Can you work these out from the model? Positions are in its coordinate system, mm. Face numbers are marked on the shaded views. A direction names the side the tool comes from. Give positions to 0.01 mm unless a question says otherwise; leave off trailing zeros. Order: outer loops, then holes, each group sorted by start corner. A loop starts at its lowest first (then second) coordinate and runs counter-clockwise, first axis right, second up.
Item 1: I want a section at B-B, the plane x = -2. Write out the boundary of the cut face in (y, z).
Item 2: I want a section at A-A, the plane z = 6.5. Write out the boundary of the cut face in (x, y), then the cut area to 3 significant figures.
Item 3: I want a section at C-C, the plane y = -11.25. Write out the boundary of the cut face in (x, z), then the cut area to 3 significant figures.
Item 4: I want a section at D-D, the plane z = 0. Count the separate pieces of the cut face and the enclosed holes in it, then the cut area to 3 significant figures.
Item 5: Which directions (+Z, -Z, +X, -X, +Y, -Y) give clear straight access to the entire face, cutting with the end or side of a thin tool? Please do the marked faces 5 and 6.
Item 6: I'm going to push flat-ended pins straight in: pin 1 Ø2.5 at (x, z) = (13, -0.5) entering from -Y; pin 2 Ø3 at (x, z) = (31.75, 0) entering from +Y; pin 3 Ø1.9 at (y, z) = (-10, -1.5) entering from -X; pin 4 Ø1 at (y, z) = (-9, -3.5) entering from +X. Where does each tip first touch, or does it pass through?
Item 7: If we mould it in two halves opening along X, with no side actions, what happens to the marked faces 1, 2, 3 and 4? For each: +X half, -X half, draft (parallel to the pull), parting line (faces both ways), or undercut.
Item 8: If I drill on line 1 along X through (y, z) = (-9.25, 0); line 2 along X through (y, z) = (-4.5, 0); line 3 along X through (y, z) = (-10.5, -5), over which ranges is the centre line in solid material (lowest first)?
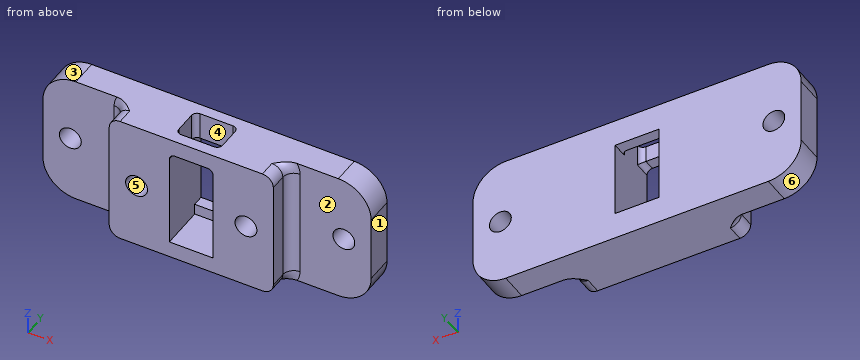
```python
from build123d import *

# Parameters (mm, degrees)
SKETCH1_W           = 38.1
SKETCH1_H           = 30.48
SKETCH1_R           = 2.54
SKETCH1_W_2         = 10.16
SKETCH1_H_2         = 22.86
BOSS_EXTRUDE1_DEPTH = 12.7
SKETCH2_W           = 10.16
SKETCH2_H           = 2.54
BOSS_EXTRUDE2_DEPTH = 2.54
SKETCH3_W           = 10.16
SKETCH3_H           = 2.54
BOSS_EXTRUDE3_DEPTH = 2.54
FILLET1_R           = 2.54
SKETCH4_W           = 10.16
SKETCH4_H           = 7.62
CUT_EXTRUDE1_DEPTH  = 36.149415358
FILLET2_R           = 1.27
BOSS_EXTRUDE4_START = -6.35
SKETCH5_R           = 2.54
BOSS_EXTRUDE4_DEPTH = 6.35
SKETCH6_R           = 2.54
CUT_EXTRUDE2_DEPTH  = 43.955297694
FILLET3_R           = 7.62
FILLET4_R           = 2.54


with BuildPart() as part:
    # Sketch1 → Boss-Extrude1 (new body)
    with BuildSketch(Plane(origin=(0, 0, 0), x_dir=(1, 0, 0), z_dir=(0, 1, 0))):
        Rectangle(SKETCH1_W, SKETCH1_H)
        with Locations(Location((12.7, 0, 0), (0, 0, 270))):
            Circle(SKETCH1_R, mode=Mode.SUBTRACT)
        with Locations(Location((-12.7, 0, 0), (0, 0, 270))):
            Circle(SKETCH1_R, mode=Mode.SUBTRACT)
        Rectangle(SKETCH1_W_2, SKETCH1_H_2, mode=Mode.SUBTRACT)
    extrude(amount=-BOSS_EXTRUDE1_DEPTH)

    # Sketch2 → Boss-Extrude2 (add)
    with BuildSketch(Plane.XY.offset(-11.43)):
        with Locations((0, -1.27)):
            Rectangle(SKETCH2_W, SKETCH2_H)
    extrude(amount=BOSS_EXTRUDE2_DEPTH)

    # Sketch3 → Boss-Extrude3 (add)
    with BuildSketch(Plane(origin=(0, 0, 11.43), x_dir=(-1, 0, 0), z_dir=(0, 0, -1))):
        with Locations((0, -1.27)):
            Rectangle(SKETCH3_W, SKETCH3_H)
    extrude(amount=BOSS_EXTRUDE3_DEPTH)

    # Fillet1
    fillet1_edges = [part.edges().sort_by_distance(p)[0] for p in [
        (19.05, -6.35, 15.24),
        (-19.05, -6.35, 15.24),
        (-19.05, -6.35, -15.24),
        (19.05, -6.35, -15.24),
    ]]
    fillet(fillet1_edges, radius=FILLET1_R)

    # Sketch4 → Cut-Extrude1 (cut, through all)
    with BuildSketch(Plane(origin=(0, 0, 11.43), x_dir=(-1, 0, 0), z_dir=(0, 0, -1))):
        with Locations((0, -6.35)):
            Rectangle(SKETCH4_W, SKETCH4_H)
    extrude(amount=-CUT_EXTRUDE1_DEPTH, mode=Mode.SUBTRACT)

    # Fillet2
    fillet2_edges = [part.edges().sort_by_distance(p)[0] for p in [
        (-5.08, -11.43, 11.43),
        (5.08, -11.43, 11.43),
        (-5.08, -2.54, 12.065),
        (5.08, -2.54, 12.065),
        (5.08, -10.16, 13.335),
        (-5.08, -10.16, 13.335),
    ]]
    fillet(fillet2_edges, radius=FILLET2_R)

    # Sketch5 → Boss-Extrude4 (add)
    with BuildSketch(Plane(origin=(0, 0, 0), x_dir=(1, 0, 0), z_dir=(0, 1, 0)).offset(BOSS_EXTRUDE4_START)):
        with BuildLine():
            Line((-16.51, 15.24), (-38.1, 15.24))
            Line((-38.1, 15.24), (-38.1, -15.24))
            Line((-38.1, -15.24), (-16.51, -15.24))
            ThreePointArc((-16.51, -15.24), (-18.306051224, -14.496051224), (-19.05, -12.7))
            Line((-19.05, -12.7), (-19.05, 12.7))
            ThreePointArc((-19.05, 12.7), (-18.306051224, 14.496051224), (-16.51, 15.24))
        make_face()
        with BuildLine():
            Line((38.1, 15.24), (16.51, 15.24))
            ThreePointArc((16.51, 15.24), (18.306051224, 14.496051224), (19.05, 12.7))
            Line((19.05, 12.7), (19.05, -12.7))
            ThreePointArc((19.05, -12.7), (18.306051224, -14.496051224), (16.51, -15.24))
            Line((16.51, -15.24), (38.1, -15.24))
            Line((38.1, -15.24), (38.1, 15.24))
        make_face()
        with Locations(Location((12.7, 0, 0), (0, 0, 270))):
            Circle(SKETCH5_R)
        with Locations(Location((-12.7, 0, 0), (0, 0, 270))):
            Circle(SKETCH5_R)
    extrude(amount=BOSS_EXTRUDE4_DEPTH)

    # Sketch6 → Cut-Extrude2 (cut, through all)
    with BuildSketch(Plane(origin=(0, 0, 0), x_dir=(1, 0, 0), z_dir=(0, 1, 0))):
        with Locations(Location((-31.75, 0, 0), (0, 0, 270))):
            Circle(SKETCH6_R)
        with Locations(Location((31.75, 0, 0), (0, 0, 270))):
            Circle(SKETCH6_R)
    extrude(amount=-CUT_EXTRUDE2_DEPTH, mode=Mode.SUBTRACT)

    # Fillet3
    fillet3_edges = [part.edges().sort_by_distance(p)[0] for p in [
        (38.1, -3.175, 15.24),
        (-38.1, -3.175, 15.24),
        (-38.1, -3.175, -15.24),
        (38.1, -3.175, -15.24),
    ]]
    fillet(fillet3_edges, radius=FILLET3_R)

    # Fillet4
    # the kernel refuses this fillet: 2.54 mm, written as the material it adds along each edge
    with BuildSketch(Plane(origin=(-16.51, -6.35, -12.7), x_dir=(-1, 0, 0), z_dir=(0, 0, 1))) as fillet4_piece_1_section:
        with BuildLine():
            CenterArc((2.54 + FILLET4_R, FILLET4_R), FILLET4_R, 180, 90)
            Line((2.54, FILLET4_R), (2.54, 0))
            Line((2.54, 0), (2.54 + FILLET4_R, 0))
        make_face()
    fillet4_piece_1 = revolve(axis=Axis((-16.51, -6.35, -12.7), (0, -1, 0)), revolution_arc=233.296989237, mode=Mode.PRIVATE)
    fillet4_piece_1 = split(fillet4_piece_1, bisect_by=Plane(origin=(-19.608229137, -6.77494251, -15.24), z_dir=(0, 0, 1)), keep=Keep.TOP, mode=Mode.PRIVATE)
    add(fillet4_piece_1)
    with BuildSketch(Plane(origin=(16.51, -6.35, 12.7), x_dir=(1, 0, 0), z_dir=(0, 0, -1))) as fillet4_piece_2_section:
        with BuildLine():
            CenterArc((2.54 + FILLET4_R, FILLET4_R), FILLET4_R, 180, 90)
            Line((2.54, FILLET4_R), (2.54, 0))
            Line((2.54, 0), (2.54 + FILLET4_R, 0))
        make_face()
    fillet4_piece_2 = revolve(axis=Axis((16.51, -6.35, 12.7), (0, -1, 0)), revolution_arc=233.296989237, mode=Mode.PRIVATE)
    fillet4_piece_2 = split(fillet4_piece_2, bisect_by=Plane(origin=(19.608229137, -6.77494251, 15.24), z_dir=(0, 0, -1)), keep=Keep.TOP, mode=Mode.PRIVATE)
    add(fillet4_piece_2)
    with BuildSketch(Plane(origin=(-16.51, -6.35, 12.7), x_dir=(0.5976672776328222, 0, -0.8017442392976523), z_dir=(-0.8017442392976523, 0, -0.5976672776328222))) as fillet4_piece_3_section:
        with BuildLine():
            CenterArc((2.54 + FILLET4_R, FILLET4_R), FILLET4_R, 180, 90)
            Line((2.54, FILLET4_R), (2.54, 0))
            Line((2.54, 0), (2.54 + FILLET4_R, 0))
        make_face()
    fillet4_piece_3 = revolve(axis=Axis((-16.51, -6.35, 12.7), (0, -1, 0)), revolution_arc=233.296989237, mode=Mode.PRIVATE)
    fillet4_piece_3 = split(fillet4_piece_3, bisect_by=Plane(origin=(-18.414845025, -7.141535935, 15.24), z_dir=(0, 0, -1)), keep=Keep.TOP, mode=Mode.PRIVATE)
    add(fillet4_piece_3)
    with BuildSketch(Plane(origin=(-19.05, -6.35, 12.7), x_dir=(-1, 0, 0), z_dir=(0, 0, -1)), Plane(origin=(19.05, -6.35, -12.7), x_dir=(1, 0, 0), z_dir=(0, 0, 1))) as fillet4_piece_4:
        with BuildLine():
            CenterArc((FILLET4_R, -FILLET4_R), FILLET4_R, 90, 90)
            Line((0, -FILLET4_R), (0, 0))
            Line((0, 0), (FILLET4_R, 0))
        make_face()
    extrude(amount=25.4)
    with BuildSketch(Plane(origin=(16.51, -6.35, -12.7), x_dir=(-0.5976672776328322, 0, 0.8017442392976448), z_dir=(0.8017442392976448, 0, 0.5976672776328322))) as fillet4_piece_5_section:
        with BuildLine():
            CenterArc((2.54 + FILLET4_R, FILLET4_R), FILLET4_R, 180, 90)
            Line((2.54, FILLET4_R), (2.54, 0))
            Line((2.54, 0), (2.54 + FILLET4_R, 0))
        make_face()
    fillet4_piece_5 = revolve(axis=Axis((16.51, -6.35, -12.7), (0, -1, 0)), revolution_arc=233.296989237, mode=Mode.PRIVATE)
    fillet4_piece_5 = split(fillet4_piece_5, bisect_by=Plane(origin=(18.414845035, -7.141535946, -15.24), z_dir=(0, 0, 1)), keep=Keep.TOP, mode=Mode.PRIVATE)
    add(fillet4_piece_5)


solid = part.part
```
Results list:
1. outline: (-12.7, -15.24) - (0, -15.24) - (0, -8.89) - (-2.54, -8.89) - (-2.54, -11.43) - (-12.7, -11.43) - close; (-12.7, 11.43) - (-10.16, 11.43) - (-10.16, 15.24) - (-12.7, 15.24) - close; (-2.54, 8.89) - (0, 8.89) - (0, 15.24) - (-2.54, 15.24) - close
2. outline: (-38.1, -6.35) - (-21.59, -6.35) arc R2.54 cw to (-19.05, -8.89) - (-19.05, -12.7) - (-5.08, -12.7) - (-5.08, 0) - (-38.1, 0) - close; (5.08, -12.7) - (19.05, -12.7) - (19.05, -8.89) arc R2.54 cw to (21.59, -6.35) - (38.1, -6.35) - (38.1, 0) - (5.08, 0) - close
2. area: 600 mm2
3. outline: (-19.05, -12.7) arc R2.54 ccw to (-16.51, -15.24) - (16.51, -15.24) arc R2.54 ccw to (19.05, -12.7) - (19.05, 12.7) arc R2.54 ccw to (16.51, 15.24) - (-16.51, 15.24) arc R2.54 ccw to (-19.05, 12.7) - close; hole circle Ø5.08 at (-12.7, 0); hole (-5.08, -11.43) - (5.08, -11.43) - (5.08, 10.16) arc R1.27 ccw to (3.81, 11.43) - (-3.81, 11.43) arc R1.27 ccw to (-5.08, 10.16) - close; hole circle Ø5.08 at (12.7, 0)
3. area: 884 mm2
4. separate pieces: 4
4. enclosed holes: 0
4. area: 471 mm2
5. face 5: -Y
5. face 6: -Z, -X, +Y, -Y
6. pin 1: stops at y = -6.35
6. pin 2: passes through
6. pin 3: stops at x = -19.05
6. pin 4: stops at x = 19.08
7. face 1: +X half
7. face 2: draft
7. face 3: -X half
7. face 4: undercut
8. line 1: x = -19.05 to -15.24, -10.16 to -5.08, 5.08 to 10.16, 15.24 to 19.05
8. line 2: x = -38.1 to -34.29, -29.21 to -5.08, 5.08 to 29.21, 34.29 to 38.1
8. line 3: x = -19.05 to -5.08, 5.08 to 19.05
